Geometry: final body of the model. Coordinates: model frame, mm. A direction names the side the tool comes from. Coordinates: 2 decimals unless noted, no trailing zeros. Order: outer loops, then holes, each group sorted by start corner. A loop starts at its lowest first (then second) coordinate and runs counter-clockwise, first axis right, second up. Notation, with made-up numbers: (-6.75, -11) -> (47.25, -11) arc R20 ccw to (47.25, 6) -> close; hole circle Ø11 at (21, 9). An arc over 180 degrees is marked (long way). Answer in a Markdown table with one row per item. Add a question column.
1) Section query B-B on y = -37. Return the cut outline in (x, z).
2) Ray query, line 1 (Y direction, x = 88, z = 2.65); line 2 (Y direction, x = 35, z = 2.8); line 3 (Y direction, x = 32, z = 1.85). Return the intervals inside material, ascending. Write a range as from..to.
3) Pull-direction query (X, two-part tool) for faces 1 (the face through (0, -51, 2)), 2 (the face through (49, -49, 0)), 3 (the face through (93, -13, 2)), 4 (the face through (85, -40, 2)); classes: +X half, -X half, draft (parallel to the pull), parting line (faces both ways), or undercut.
4) Section query A-A on x = 35. Return the cut outline in (y, z).
5) Contact query for flat-ended pins moving along their axis: P1, Ø1.5, axis at x = 85, z = 2.5, coming from the +Y side; P2, Ø7, axis at x = 35, y = -55, coming from the -Z side. Output: stop coordinate, or through.
6) Set-up query: faces 5 (the face through (77, -37, 2)), 6 (the face through (100, -51, 2)). Return all of +Z, -Z, +X, -X, +Y, -Y with unobstructed straight access to the full face (end or side cutting, diameter ignored); none if empty.
7) Section query C-C on z = 1.15. Return the cut outline in (x, y), then the cut area to 3 significant figures.
```python
from build123d import *

# Parameters (mm, degrees)
ESQUISSE1_W             = 100
ESQUISSE1_H             = 100
BOSS_EXTRU_1_DEPTH      = 5
ESQUISSE2_R             = 6
ENL_V_MAT_EXTRU_1_DEPTH = 5


with BuildPart() as part:
    # Esquisse1 → Boss.-Extru.1 (new body)
    with BuildSketch(Plane.XY):
        with Locations((50, -50)):
            Rectangle(ESQUISSE1_W, ESQUISSE1_H)
        with BuildLine():
            Line((80, -10), (90, -10))
            ThreePointArc((90, -10), (93, -13), (90, -16))
            Line((90, -16), (80, -16))
            ThreePointArc((80, -16), (77, -13), (80, -10))
        make_face(mode=Mode.SUBTRACT)
        with BuildLine():
            Line((80, -34), (90, -34))
            ThreePointArc((90, -34), (93, -37), (90, -40))
            Line((90, -40), (80, -40))
            ThreePointArc((80, -40), (77, -37), (80, -34))
        make_face(mode=Mode.SUBTRACT)
    extrude(amount=BOSS_EXTRU_1_DEPTH)

    # Esquisse2 → Enlèv. mat.-Extru.1 (cut)
    with BuildSketch(Plane.XY.offset(5)):
        with Locations((35, -55)):
            Circle(ESQUISSE2_R)
    extrude(amount=-ENL_V_MAT_EXTRU_1_DEPTH, mode=Mode.SUBTRACT)


solid = part.part
```
Result:
| question | item | result |
|---|---|---|
| 1 | outline | (0, 0) -> (77, 0) -> (77, 5) -> (0, 5) -> close; (93, 0) -> (100, 0) -> (100, 5) -> (93, 5) -> close |
| 2 | line 1 | -100..-40, -34..-16, -10..0 |
| 2 | line 2 | -100..-61, -49..0 |
| 2 | line 3 | -100..-60.2, -49.8..0 |
| 3 | face 1 | -X half |
| 3 | face 2 | draft |
| 3 | face 3 | undercut |
| 3 | face 4 | undercut |
| 4 | outline | (-100, 0) -> (-61, 0) -> (-61, 5) -> (-100, 5) -> close; (-49, 0) -> (0, 0) -> (0, 5) -> (-49, 5) -> close |
| 5 | P1 | y = 0 |
| 5 | P2 | through |
| 6 | face 5 | +Z, -Z |
| 6 | face 6 | +Z, -Z, +X, +Y, -Y |
| 7 | outline | (0, -100) -> (100, -100) -> (100, 0) -> (0, 0) -> close; hole circle Ø12 at (35, -55); hole (80, -40) -> (90, -40) arc R3 ccw to (90, -34) -> (80, -34) arc R3 ccw to start; hole (80, -16) -> (90, -16) arc R3 ccw to (90, -10) -> (80, -10) arc R3 ccw to start |
| 7 | area | 9,710 mm2 |
